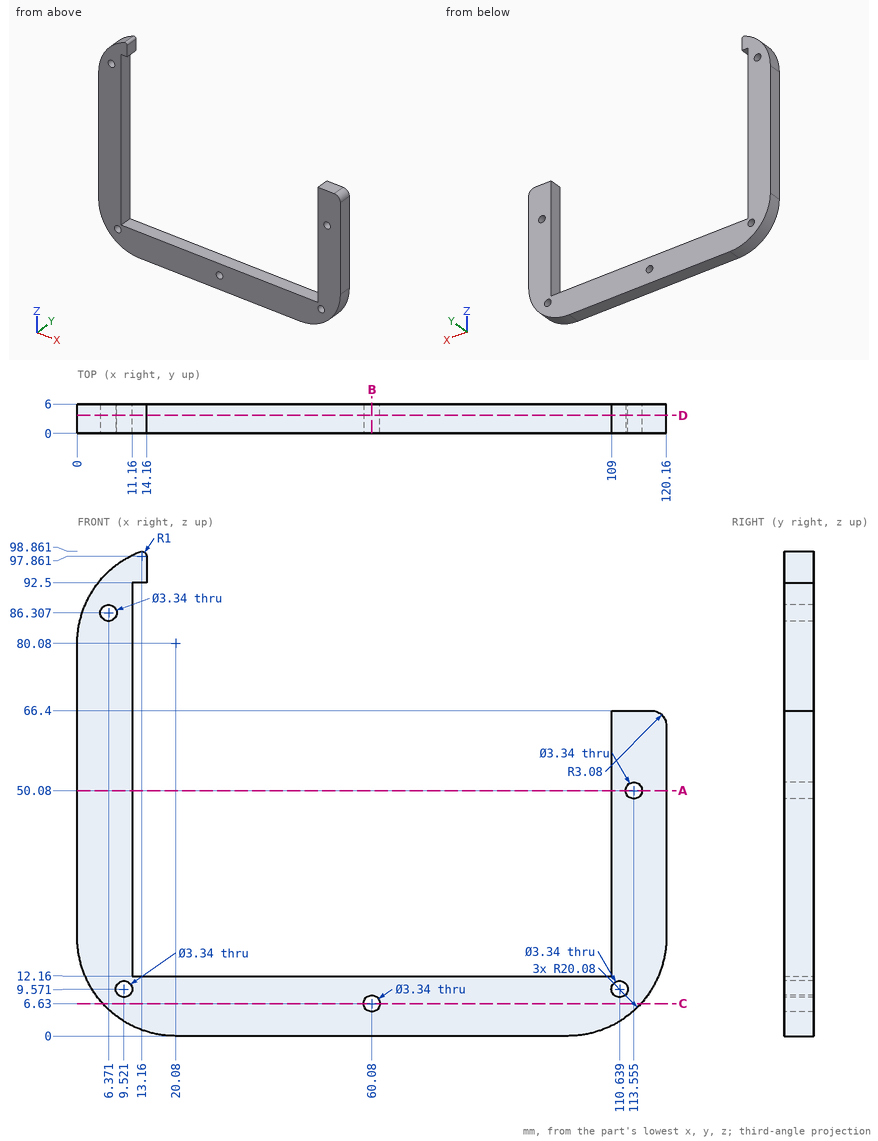
Answer from the drawing. Dimensions are ordinates in mm from the lowest x, y and z of the part. Round coordinates to 2 decimals unless told otherwise and drop trailing zeros. Write each loop counter-clockwise with the first axis right and the second up, starting at its lowest first coordinate (ties: lowest second). Pieces come first, ordered by that corner, then holes. Notation, with made-up numbers: (69.5, -26) -> (86.5, -26) arc R21 cw to (86.5, 12) -> close; hole circle Ø6 at (5, 66.5). An arc over 180 degrees is marked (long way). Answer in a Markdown table with one row per item. Add a question column.
1) Given P1, Ø3, axis at y = 3, z = 72.5, coming from the +X side; P2, Ø1.8, axis at x = 111.5, y = 4, coming from the +Z side; P3, Ø1.5, axis at x = 100, y = 3, coming from the +Z side; P4, Ø2, axis at x = 9.52, z = 9.57, coming from the +Y side, each flat-ended and moving along its own axis, determine where each tip first touches the part or whether it passes through.
2) Find section A-A, the plane z = 50.08. Determine the outline of the cut face in (x, y) (1 decimal), and give its area (3 significant figures).
3) Find section B-B, the plane x = 60.08. Determine the outline of the cut face in (y, z).
4) Find section C-C, the plane z = 6.63. Determine the outline of the cut face in (x, y).
5) Consider line 1 (Z direction, x = 60.08, y = 3.4); line 2 (X direction, y = 4.55, z = 47.5); line 3 (X direction, y = 5.7, z = 67.5). Determine where each line is inside the solid, lowest interval first.
6) Find section D-D, the plane y = 3.7. State how many separate pieces and enclosed holes the cut face has, and give its area (3 significant figures).
Findings below:
| question | item | result |
|---|---|---|
| 1 | P1 | x = 11.16 |
| 1 | P2 | z = 66.4 |
| 1 | P3 | z = 12.16 |
| 1 | P4 | through |
| 2 | outline | (0, 0) -> (11.2, 0) -> (11.2, 6) -> (0, 6) -> close; (109, 0) -> (111.9, 0) -> (111.9, 6) -> (109, 6) -> close; (115.2, 0) -> (120.2, 0) -> (120.2, 6) -> (115.2, 6) -> close |
| 2 | area | 114 mm² |
| 3 | outline | (0, 0) -> (6, 0) -> (6, 4.96) -> (0, 4.96) -> close; (0, 8.3) -> (6, 8.3) -> (6, 12.16) -> (0, 12.16) -> close |
| 4 | outline | (5.17, 0) -> (58.41, 0) -> (58.41, 6) -> (5.17, 6) -> close; (61.75, 0) -> (114.99, 0) -> (114.99, 6) -> (61.75, 6) -> close |
| 5 | line 1 | 0 to 4.96, 8.3 to 12.16 |
| 5 | line 2 | 0 to 11.16, 109 to 120.16 |
| 5 | line 3 | 0 to 11.16 |
| 6 | separate pieces | 1 |
| 6 | enclosed holes | 5 |
| 6 | area | 2,770 mm² |
